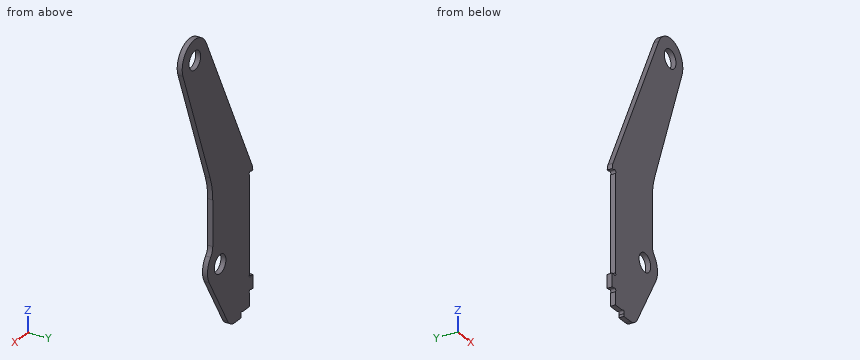
from build123d import *

# Parameters (mm, degrees)
F0_R     = 8.73125
F1_DEPTH = 4.7625
F2_W     = 4.7625
F2_H     = 12.7
F3_DEPTH = 4.7625
F4_R     = 1.5875
F5_DEPTH = 4.7635


with BuildPart() as f1:
    # F0 (on Front) → F1 (new body)
    with BuildSketch(Plane.XZ):
        with BuildLine():
            Line((-49.2125, 63.5), (-44.45, 63.5))
            Line((-44.45, 63.5), (-44.45, -58.7375))
            Line((-44.45, -58.7375), (-31.75, -58.7375))
            Line((-31.75, -58.7375), (-31.75, -63.5))
            Line((-31.75, -63.5), (-22.225, -63.5))
            ThreePointArc((-22.225, -63.5), (-15.894715, -61.809881), (-11.249301, -57.189368))
            Line((-11.249301, -57.189368), (16.463549, -9.584053))
            ThreePointArc((16.463549, -9.584053), (18.959012, 1.85967), (14.2875, 12.600391))
            ThreePointArc((14.2875, 12.600391), (11.932738, 16.510523), (11.1125, 21.000651))
            Line((11.1125, 21.000651), (11.1125, 63.5))
            ThreePointArc((11.1125, 63.5), (12.098669, 74.647689), (15.026546, 85.449126))
            Line((15.026546, 85.449126), (55.975786, 196.615262))
            ThreePointArc((55.975786, 196.615262), (45.548054, 220.733653), (20.950146, 211.493672))
            Line((20.950146, 211.493672), (-47.945736, 69.029115))
            ThreePointArc((-47.945736, 69.029115), (-48.891759, 66.336186), (-49.2125, 63.5))
        make_face()
        Circle(F0_R, mode=Mode.SUBTRACT)
        with Locations((38.1, 203.2)):
            Circle(F0_R, mode=Mode.SUBTRACT)
    extrude(amount=F1_DEPTH)

    # F2 (on Front) → F3 (join, through all)
    with BuildSketch(Plane.XZ):
        with Locations((-46.83125, -38.1)):
            Rectangle(F2_W, F2_H)
    extrude(amount=F3_DEPTH)

    # F4 (on Front) → F5 (cut, through all)
    with BuildSketch(Plane.XZ):
        with Locations((-45.392927, 62.557073)):
            Circle(F4_R)
        with Locations((-32.692927, -59.680427)):
            Circle(F4_R)
        with Locations((-45.392927, -45.392927)):
            Circle(F4_R)
        with Locations((-45.392927, -30.807073)):
            Circle(F4_R)
    extrude(amount=F5_DEPTH, mode=Mode.SUBTRACT)


solid = f1.part
Geometry: final body of the model. Coordinates: model frame, mm. Give positions to 0.01 mm unless a question says otherwise; leave off trailing zeros. Write each loop counter-clockwise with the first axis right and the second up, starting at its lowest first coordinate (ties: lowest second). Pieces come first, ordered by that corner, then holes. Notation, with made-up numbers: M 72,-11 L 79,-11 A24 ccw 79,21 Z; hole C 58.5,80 d8. An arc over 180 degrees is marked long. Answer in a Markdown table with one row per item. Add a question column.
(1) First-contact query: pin 1 (2.5 mm diameter, centred on y = -1.5, z = -54.5, fed in from -X); pin 2 (1.5 mm diameter, centred on y = -2.5, z = 82.5, fed in from -X); pin 3 (14 mm diameter, centred on x = 0, z = 0, fed in from -Y); pin 4 (1.4 mm diameter, centred on y = -1.5, z = 42, fed in from +X). Flat tips, straight axial feed; report the tip coordinate or a pass-through.
(2) Ray query, line 1 (X direction, y = -2.75, z = 22.5); line 2 (Z direction, x = -4, y = -1.2); line 3 (Z direction, x = -15.5, y = -2.2). Return the intervals inside material, ascending.
(3) Section B-B on y = -2.9. State how many separate pieces and enclosed holes the cut face has, and give its area (3 significant figures).
(4) Section D-D on z = 30. Return loops of the section in (x, y), and give its area (3 significant figures).
(5) Section C-C on x = 38.1. Return loops of the section in (y, z), and give its area (3 significant figures).
(6) Section A-A on z = 0. Return loops of the section in (x, y), and give its area (3 significant figures).
Result set:
| question | item | result |
|---|---|---|
| 1 | pin 1 | stops at x = -44.45 |
| 1 | pin 2 | stops at x = -41.79 |
| 1 | pin 3 | passes through |
| 1 | pin 4 | stops at x = 11.11 |
| 2 | line 1 | x = -44.45 to 11.11 |
| 2 | line 2 | z = -44.74 to -7.76, 7.76 to 159.9 |
| 2 | line 3 | z = -61.57 to 136.12 |
| 3 | separate pieces | 1 |
| 3 | enclosed holes | 2 |
| 3 | area | 13,700 mm^2 |
| 4 | outline | M -44.45,-4.76 L 11.11,-4.76 L 11.11,0 L -44.45,0 Z |
| 4 | area | 265 mm^2 |
| 5 | outline | M -4.76,148.09 L 0,148.09 L 0,194.47 L -4.76,194.47 Z; M -4.76,211.93 L 0,211.93 L 0,222.25 L -4.76,222.25 Z |
| 5 | area | 270 mm^2 |
| 6 | outline | M -44.45,-4.76 L -8.73,-4.76 L -8.73,0 L -44.45,0 Z; M 8.73,-4.76 L 19.05,-4.76 L 19.05,0 L 8.73,0 Z |
| 6 | area | 219 mm^2 |
